CAD build for the part. Positions are in the model's coordinates, mm. Face numbers are marked on the shaded views. A direction names the side the tool comes from. Give positions to 0.01 mm unless a question says otherwise; leave off trailing zeros. Order: outer loops, then holes, each group sorted by start corner. A loop starts at its lowest first (then second) coordinate and runs counter-clockwise, first axis right, second up. Notation, with made-up numbers: (34.25, -31.75) -> (67.25, -31.75) arc R26 ccw to (67.25, 4.25) -> close; hole circle Ø3 at (36, 29.5). An arc over 180 degrees is marked (long way). Use one line per item in the form item = value. Start each with the question number.
1) Drop flat-ended pins along their axis: P1, Ø12, axis at y = -10, z = -22, coming from the -X side; P2, Ø1.5, axis at y = 3.5, z = -13.5, coming from the -X side; P3, Ø8, axis at y = 16.5, z = -6, coming from the +X side. Give the stop position or say it passes through.
2) Cut at C-C, the plane z = -12.25. Give the cut face in (x, y), and give its area (3 significant figures).
3) Cut at A-A, the plane x = 0. Give the cut face in (y, z).
4) Mould opens along X. For the marked faces 1, 2 and 3 say: pulls with the +X half, pulls with the -X half, needs draft (parallel to the pull), parting line crosses it, or undercut.
5) Tool access for the marked faces 4 and 5: list every direction of +Z, -Z, +X, -X, +Y, -Y with a clear straight run to the whole face (end or side of a thin tool).
6) Probe line 1 (Z direction, x = 20, y = -17); line 2 (X direction, y = -13, z = -16.5); line 3 (X direction, y = -9.5, z = -6.75). List the from-to ranges inside material, lowest first.
7) Cut at B-B, the plane z = -23. Give the cut face in (x, y), and give its area (3 significant figures).
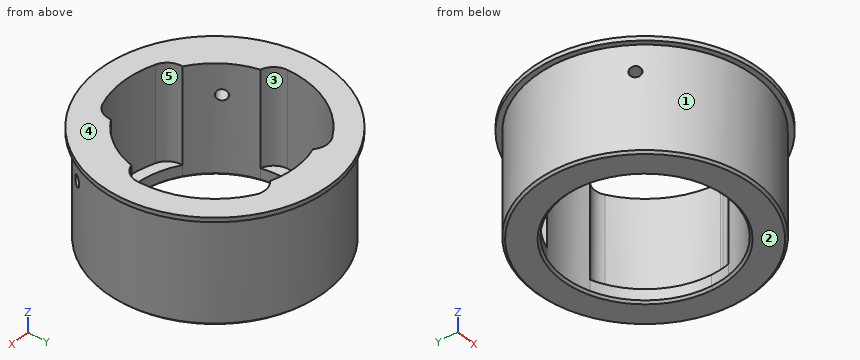
from build123d import *

# Parameters (mm, degrees)
F0_R           = 26.5
F0_R_2         = 25.3
F1_DEPTH       = 1
F2_DEPTH       = 25
F3_DEPTH       = 22
F4_T1_DEPTH    = 22
F9_D           = 2.5
F9_DEPTH       = 25
F9_START       = 1.2308984
F9_TIP         = 0.7510757738
F9_ON_F7_D     = 2.5
F9_ON_F7_DEPTH = 25
F9_ON_F7_START = 1.2308984
F9_ON_F7_TIP   = 0.7510757738
F10_SIZE       = 0.5


# Not quite as in the source:
# - a fillet or chamfer that OpenCascade refuses, or shapes differently, is made with other operations: its cross-section is extruded or revolved along the edge and cut away or added


with BuildPart() as f1:
    # F0 (on Top) → F1 (new body)
    with BuildSketch(Plane.XY):
        Circle(F0_R)
        Circle(F0_R_2, mode=Mode.SUBTRACT)
        Circle(F0_R_2)
        with BuildLine():
            ThreePointArc((-6.7924528302, 19.8711495528), (0, 21), (6.7924528302, 19.8711495528))
            ThreePointArc((6.7924528302, 19.8711495528), (17.0827619171, 12.2138955818), (21, 0))
            ThreePointArc((21, 0), (20.8522276614, -2.4868859159), (20.4109903277, -4.9387725035))
            ThreePointArc((20.4109903277, -4.9387725035), (17.0984542242, -12.1919179436), (11.320754717, -17.6872980593))
            ThreePointArc((11.320754717, -17.6872980593), (0, -21), (-11.320754717, -17.6872980593))
            ThreePointArc((-11.320754717, -17.6872980593), (-17.0984542242, -12.1919179436), (-20.4109903277, -4.9387725035))
            ThreePointArc((-20.4109903277, -4.9387725035), (-18.4089621658, 10.1049548232), (-6.7924528302, 19.8711495528))
        make_face(mode=Mode.SUBTRACT)
    extrude(amount=-F1_DEPTH)

    # F0 (on Top) → F2 (join)
    with BuildSketch(Plane.XY):
        Circle(F0_R_2)
        with BuildLine():
            ThreePointArc((-6.7924528302, 19.8711495528), (0, 21), (6.7924528302, 19.8711495528))
            ThreePointArc((6.7924528302, 19.8711495528), (17.0827619171, 12.2138955818), (21, 0))
            ThreePointArc((21, 0), (20.8522276614, -2.4868859159), (20.4109903277, -4.9387725035))
            ThreePointArc((20.4109903277, -4.9387725035), (17.0984542242, -12.1919179436), (11.320754717, -17.6872980593))
            ThreePointArc((11.320754717, -17.6872980593), (0, -21), (-11.320754717, -17.6872980593))
            ThreePointArc((-11.320754717, -17.6872980593), (-17.0984542242, -12.1919179436), (-20.4109903277, -4.9387725035))
            ThreePointArc((-20.4109903277, -4.9387725035), (-18.4089621658, 10.1049548232), (-6.7924528302, 19.8711495528))
        make_face(mode=Mode.SUBTRACT)
        with BuildLine():
            Line((20.4109903277, -4.9387725035), (18.0297081228, -4.3625823781))
            ThreePointArc((18.0297081228, -4.3625823781), (15.1036345647, -10.7695275168), (10, -15.6237799524))
            Line((10, -15.6237799524), (11.320754717, -17.6872980593))
            ThreePointArc((11.320754717, -17.6872980593), (17.0984542242, -12.1919179436), (20.4109903277, -4.9387725035))
        make_face()
        with BuildLine():
            ThreePointArc((6, 17.5528487716), (15.0897730268, 10.7889410973), (18.55, 0))
            ThreePointArc((18.55, 0), (18.4194677675, -2.1967492257), (18.0297081228, -4.3625823781))
            Line((18.0297081228, -4.3625823781), (20.4109903277, -4.9387725035))
            ThreePointArc((20.4109903277, -4.9387725035), (20.8522276614, -2.4868859159), (21, 0))
            ThreePointArc((21, 0), (17.0827619171, 12.2138955818), (6.7924528302, 19.8711495528))
            Line((6.7924528302, 19.8711495528), (6, 17.5528487716))
        make_face()
        with BuildLine():
            ThreePointArc((-6, 17.5528487716), (0, 18.55), (6, 17.5528487716))
            Line((6, 17.5528487716), (6.7924528302, 19.8711495528))
            ThreePointArc((6.7924528302, 19.8711495528), (0, 21), (-6.7924528302, 19.8711495528))
            Line((-6.7924528302, 19.8711495528), (-6, 17.5528487716))
        make_face()
        with BuildLine():
            ThreePointArc((-18.0297081228, -4.3625823781), (-16.2612499131, 8.9260434271), (-6, 17.5528487716))
            Line((-6, 17.5528487716), (-6.7924528302, 19.8711495528))
            ThreePointArc((-6.7924528302, 19.8711495528), (-18.4089621658, 10.1049548232), (-20.4109903277, -4.9387725035))
            Line((-20.4109903277, -4.9387725035), (-18.0297081228, -4.3625823781))
        make_face()
        with BuildLine():
            ThreePointArc((-10, -15.6237799524), (-15.1036345647, -10.7695275168), (-18.0297081228, -4.3625823781))
            Line((-18.0297081228, -4.3625823781), (-20.4109903277, -4.9387725035))
            ThreePointArc((-20.4109903277, -4.9387725035), (-17.0984542242, -12.1919179436), (-11.320754717, -17.6872980593))
            Line((-11.320754717, -17.6872980593), (-10, -15.6237799524))
        make_face()
        with BuildLine():
            Line((11.320754717, -17.6872980593), (10, -15.6237799524))
            ThreePointArc((10, -15.6237799524), (0, -18.55), (-10, -15.6237799524))
            Line((-10, -15.6237799524), (-11.320754717, -17.6872980593))
            ThreePointArc((-11.320754717, -17.6872980593), (0, -21), (11.320754717, -17.6872980593))
        make_face()
    extrude(amount=-F2_DEPTH)

    # F0 (on Top) → F3 (cut)
    with BuildSketch(Plane.XY):
        with BuildLine():
            ThreePointArc((6, 17.5528487716), (15.0897730268, 10.7889410973), (18.55, 0))
            ThreePointArc((18.55, 0), (18.4194677675, -2.1967492257), (18.0297081228, -4.3625823781))
            Line((18.0297081228, -4.3625823781), (20.4109903277, -4.9387725035))
            ThreePointArc((20.4109903277, -4.9387725035), (20.8522276614, -2.4868859159), (21, 0))
            ThreePointArc((21, 0), (17.0827619171, 12.2138955818), (6.7924528302, 19.8711495528))
            Line((6.7924528302, 19.8711495528), (6, 17.5528487716))
        make_face()
        with BuildLine():
            Line((11.320754717, -17.6872980593), (10, -15.6237799524))
            ThreePointArc((10, -15.6237799524), (0, -18.55), (-10, -15.6237799524))
            Line((-10, -15.6237799524), (-11.320754717, -17.6872980593))
            ThreePointArc((-11.320754717, -17.6872980593), (0, -21), (11.320754717, -17.6872980593))
        make_face()
        with BuildLine():
            ThreePointArc((-18.0297081228, -4.3625823781), (-16.2612499131, 8.9260434271), (-6, 17.5528487716))
            Line((-6, 17.5528487716), (-6.7924528302, 19.8711495528))
            ThreePointArc((-6.7924528302, 19.8711495528), (-18.4089621658, 10.1049548232), (-20.4109903277, -4.9387725035))
            Line((-20.4109903277, -4.9387725035), (-18.0297081228, -4.3625823781))
        make_face()
    extrude(amount=-F3_DEPTH, mode=Mode.SUBTRACT)

    # F4: fillet of radius 4 on 6 edges, made by hand

    # F4_s2 → F4_t1 (join)
    with BuildSketch(Plane.XY.offset(-22)):
        with BuildLine():
            ThreePointArc((10.7499670552, 18.0399059951), (8.2943373762, 18.582869286), (6, 17.5528487716))
            Line((6, 17.5528487716), (5.9459529143, 17.6118310786))
            ThreePointArc((5.9459529143, 17.6118310786), (6.3205267978, 18.737875173), (6.7167532128, 19.8970255636))
            Line((6.7167532128, 19.8970255636), (6.818328841, 19.9468491701))
            ThreePointArc((6.818328841, 19.9468491701), (8.852466778, 19.1311325317), (10.7909193107, 18.1086294465))
            Line((10.7909193107, 18.1086294465), (10.7499670552, 18.0399059951))
        make_face()
        with BuildLine():
            ThreePointArc((-6, 17.5528487716), (-8.2943373762, 18.582869286), (-10.7499670552, 18.0399059951))
            Line((-10.7499670552, 18.0399059951), (-10.7909193107, 18.1086294465))
            ThreePointArc((-10.7909193107, 18.1086294465), (-8.852466778, 19.1311325317), (-6.818328841, 19.9468491701))
            Line((-6.818328841, 19.9468491701), (-6.7167532128, 19.8970255636))
            ThreePointArc((-6.7167532128, 19.8970255636), (-6.3205267978, 18.737875173), (-5.9459529143, 17.6118310786))
            Line((-5.9459529143, 17.6118310786), (-6, 17.5528487716))
        make_face()
        with BuildLine():
            ThreePointArc((18.0297081228, -4.3625823781), (20.1305359874, -2.9800309182), (20.9909384883, -0.6168479392))
            Line((20.9909384883, -0.6168479392), (21.0709039683, -0.6191978361))
            ThreePointArc((21.0709039683, -0.6191978361), (20.8927389597, -2.8035439649), (20.4887464814, -4.957586875))
            Line((20.4887464814, -4.957586875), (20.3921759563, -5.0165286572))
            ThreePointArc((20.3921759563, -5.0165286572), (19.2015348538, -4.7284335945), (18.0504489955, -4.4398469638))
            Line((18.0504489955, -4.4398469638), (18.0297081228, -4.3625823781))
        make_face()
        with BuildLine():
            ThreePointArc((7.423758192, -19.6440274462), (9.3775452078, -18.0604736729), (10, -15.6237799524))
            Line((10, -15.6237799524), (10.0798058197, -15.6182093928))
            ThreePointArc((10.0798058197, -15.6182093928), (10.7277575416, -16.6124123212), (11.3881349001, -17.6441713746))
            Line((11.3881349001, -17.6441713746), (11.3638814016, -17.7546782424))
            ThreePointArc((11.3638814016, -17.7546782424), (9.4590814084, -18.8385821895), (7.4520391756, -19.7188618365))
            Line((7.4520391756, -19.7188618365), (7.423758192, -19.6440274462))
        make_face()
        with BuildLine():
            ThreePointArc((-10, -15.6237799524), (-9.3775452078, -18.0604736729), (-7.423758192, -19.6440274462))
            Line((-7.423758192, -19.6440274462), (-7.4520391756, -19.7188618365))
            ThreePointArc((-7.4520391756, -19.7188618365), (-9.4590814084, -18.8385821895), (-11.3638814016, -17.7546782424))
            Line((-11.3638814016, -17.7546782424), (-11.3881349001, -17.6441713746))
            ThreePointArc((-11.3881349001, -17.6441713746), (-10.7277575416, -16.6124123212), (-10.0798058197, -15.6182093928))
            Line((-10.0798058197, -15.6182093928), (-10, -15.6237799524))
        make_face()
        with BuildLine():
            ThreePointArc((-20.9909384883, -0.6168479392), (-20.1305359874, -2.9800309182), (-18.0297081228, -4.3625823781))
            Line((-18.0297081228, -4.3625823781), (-18.0504489955, -4.4398469638))
            ThreePointArc((-18.0504489955, -4.4398469638), (-19.2015348538, -4.7284335945), (-20.3921759563, -5.0165286572))
            Line((-20.3921759563, -5.0165286572), (-20.4887464814, -4.957586875))
            ThreePointArc((-20.4887464814, -4.957586875), (-20.8927389597, -2.8035439649), (-21.0709039683, -0.6191978361))
            Line((-21.0709039683, -0.6191978361), (-20.9909384883, -0.6168479392))
        make_face()
    extrude(amount=F4_T1_DEPTH)

    # F9
    # its depths count from where the whole tool has entered the part; down to there all is cleared
    with Locations(Plane(origin=(-21.5766208067, -15.3850393098, 0), x_dir=(0.5805675211, -0.8142121059, 0), z_dir=(-0.8142121059, -0.5805675211, 0)).offset(-F9_START)):
        with Locations((0, -7)):
            Hole(F9_D / 2, depth=F9_DEPTH)
            with Locations((0, 0, -(F9_DEPTH + F9_TIP / 2))):  # 118° drill point
                Cone(0, F9_D / 2, F9_TIP, mode=Mode.SUBTRACT)

    # F9 on F7
    # its depths count from where the whole tool has entered the part; down to there all is cleared
    with Locations(Plane(origin=(21.5766208067, -15.3850393098, 0), x_dir=(0.5805675211, 0.8142121059, 0), z_dir=(0.8142121059, -0.5805675211, 0)).offset(-F9_ON_F7_START)):
        with Locations((0, -7)):
            Hole(F9_ON_F7_D / 2, depth=F9_ON_F7_DEPTH)
            with Locations((0, 0, -(F9_ON_F7_DEPTH + F9_ON_F7_TIP / 2))):  # 118° drill point
                Cone(0, F9_ON_F7_D / 2, F9_ON_F7_TIP, mode=Mode.SUBTRACT)

    # F10
    f10_edges = [f1.edges().sort_by_distance(p)[0] for p in [
        (-10, 15.62378, -25),
        (-25.3, 0, -25),
    ]]
    chamfer(f10_edges, length=F10_SIZE)


solid = f1.part
Result:
q1.P1 = -24.98
q1.P2 = -25.15
q1.P3 = 22
q2.outline = circle Ø50.6 at (0, 0); hole (-20.99, -0.62) arc R4 ccw to (-18.03, -4.36) arc R18.55 ccw to (-10, -15.62) arc R4 ccw to (-7.42, -19.64) arc R21 ccw to (7.42, -19.64) arc R4 ccw to (10, -15.62) arc R18.55 ccw to (18.03, -4.36) arc R4 ccw to (20.99, -0.62) arc R21 ccw to (10.75, 18.04) arc R4 ccw to (6, 17.55) arc R18.55 ccw to (-6, 17.55) arc R4 ccw to (-10.75, 18.04) arc R21 ccw to start
q2.area = 750 mm²
q3.outline = (-26.5, -1) -> (-25.3, -1) -> (-25.3, -24.5) -> (-24.8, -25) -> (-19.05, -25) -> (-18.55, -24.5) -> (-18.55, -22) -> (-21, -22) -> (-21, 0) -> (-26.5, 0) -> close; (18.55, -24.5) -> (19.05, -25) -> (24.8, -25) -> (25.3, -24.5) -> (25.3, -1) -> (26.5, -1) -> (26.5, 0) -> (18.55, 0) -> close
q4.face_1 = parting line crosses it
q4.face_2 = needs draft
q4.face_3 = undercut
q5.face_4 = +Z, +X, -X, +Y, -Y
q5.face_5 = +Z
q6.line_1 = -1 to 0
q6.line_2 = -21.7 to -13.23, 13.23 to 21.7
q6.line_3 = -23.45 to -15.93, 15.93 to 23.45
q7.outline = circle Ø50.6 at (0, 0); hole circle Ø37.1 at (0, 0)
q7.area = 930 mm²
